from build123d import *

# Parameters (mm, degrees)
SKETCH1_R           = 2.6
BOSS_EXTRUDE1_DEPTH = 1.8
SKETCH2_R           = 2
BOSS_EXTRUDE2_DEPTH = 2.4
SKETCH3_R           = 2.35
BOSS_EXTRUDE3_DEPTH = 1
CHAMFER1_SIZE       = 0.75
CHAMFER1_SIZE2      = 0.832959386
FILLET1_R           = 0.2
SCALE1_SCALE        = 1.15


with BuildPart() as part:
    # Sketch1 → Boss-Extrude1 (new body)
    with BuildSketch(Plane(origin=(0, 0, 0), x_dir=(1, 0, 0), z_dir=(0, 1, 0))):
        Circle(SKETCH1_R)
    extrude(amount=BOSS_EXTRUDE1_DEPTH)

    # Sketch2 → Boss-Extrude2 (add)
    with BuildSketch(Plane(origin=(0, 1.8, 0), x_dir=(1, 0, 0), z_dir=(0, 1, 0))):
        Circle(SKETCH2_R)
    extrude(amount=BOSS_EXTRUDE2_DEPTH)

    # Sketch3 → Boss-Extrude3 (add)
    with BuildSketch(Plane(origin=(0, 4.2, 0), x_dir=(1, 0, 0), z_dir=(0, 1, 0))):
        Circle(SKETCH3_R)
    extrude(amount=BOSS_EXTRUDE3_DEPTH)

    # Chamfer1
    chamfer1_edges = [part.edges().sort_by_distance(p)[0] for p in [
        (-2.35, 5.2, 0),
    ]]
    chamfer1_side = [part.faces().sort_by_distance(p)[0] for p in [
        (-2.35, 4.7, 0),
    ]]
    chamfer(chamfer1_edges, length=CHAMFER1_SIZE, length2=CHAMFER1_SIZE2, reference=chamfer1_side[0])

    # Fillet1
    fillet1_edges = [part.edges().sort_by_distance(p)[0] for p in [
        (-1.517040614, 5.2, 0),
        (-2.35, 4.45, 0),
        (-2, 1.8, 0),
    ]]
    fillet(fillet1_edges, radius=FILLET1_R)


with BuildPart() as part_1:
    # Scale1: scaled about (-4.2e-08, 2.280257944, 0)
    add(part.part.scale(SCALE1_SCALE).moved(Location((6e-09, -0.342038692, 0))))


solid = part_1.part
Could you check a few things on this model? Use its own coordinates, in mm. Round coordinates to 2 decimals unless told otherwise and drop trailing zeros. Loops run counter-clockwise (first coordinate to the right, second up) from the corner with the lowest first, then second, coordinate; pieces in that order, holes last. Notation, with made-up numbers: (-9, 14.5) - (-2, 14.5) arc R25 ccw to (-2, 38.5) - close; hole circle Ø11 at (70, 50). An arc over 180 degrees is marked (long way). Write item = value, one per line.
1) Imagine slicing it at A-A (y = 4.15). Please give me the cut outline in (x, z), and give its area (3 significant figures).
Computed:
outline = circle Ø4.6 at (0, 0)
area = 16.6 mm2
2) I need wall thicknesses on line 1 along X through (y, z) = (2.35, -0.1); line 2 along Y through (x, z) = (-2.4, -0.6); line 3 along Y through (x, z) = (-1.15, -2.6). Which ranges of each line are inside material? Lowest first, please. Write a range as from..to.
Computed:
line_1 = -2.3..2.3
line_2 = -0.34..1.73, 4.49..4.98
line_3 = -0.34..1.73
3) If we mould it in two halves opening along Y, with no side actions, what happens to faces 1 (the cylindrical face through (-2.298, 3.205, -0.101)), 2 (the flat face through (0, -0.342, 0)), 3 (the cylindrical face through (-0.65, 0.68, 2.92))? For each: pulls with the +Y half, pulls with the -Y half, needs draft (parallel to the pull), parting line crosses it, or undercut.
Computed:
face_1 = undercut
face_2 = pulls with the -Y half
face_3 = needs draft
4) Imagine slicing it at B-B (y = 0.9). Please give me the cut outline in (x, z).
Computed:
outline = circle Ø5.98 at (0, 0)
5) I'm going to push flat-ended pins straight in: P1, Ø2, axis at x = -1.5, y = 1, coming from the +Z side; P2, Ø2, axis at y = 5, z = -2, coming from the -X side. Where does each tip first touch, or does it pass through?
Computed:
P1 = 2.95
P2 = -2.49
